The listing builds one solid part. Answer for the finished solid, in the listing's coordinates (mm). A direction names the side the tool comes from. Give positions to 0.01 mm unless a question says otherwise; leave off trailing zeros. Loops run counter-clockwise (first coordinate to the right, second up) from the corner with the lowest first, then second, coordinate; pieces in that order, holes last. Notation, with made-up numbers: M 80.5,-6.5 L 129.5,-6.5 A31 ccw 129.5,30.5 Z; hole C 65.5,78.25 d8. An arc over 180 degrees is marked long. One line per item, written item: value. Start each with the question number.
Q1. For faces 5 (the flat face through (6.9, 16, 6)), 6 (the cylindrical face through (6.59, 33.89, 6.45)), 7 (the cylindrical face through (6.615, 0.301, 7.056)), determine the directions among +Z, -Z, +X, -X, +Y, -Y from which every point of the face is accessible in a straight line to the end or side of a thin tool.
Q2. A cutting plane is placed at B-B, the plane y = 12. Determine the outline of the cut face in (x, z).
Q3. Consider L1, parallel to Y at x = 20, z = 1; L2, parallel to X at y = 14.5, z = 2.5; L3, parallel to Z at x = 10, y = 4. Determine where each line is inside the solid, lowest interval first.
Q4. A cutting plane is placed at C-C, the plane z = 2.5. Determine the outline of the cut face in (x, y), and give its area (3 significant figures).
Q5. A flat-ended cylindrical pin translates along its axis: pin 1 (5.5 mm diameter, centred on y = 23.5, z = 6, fed in from +X). Find the tip coordinate at first contact, or state that the pin passes through.
Q6. A cutting plane is placed at A-A, the plane x = 20. Determine the outline of the cut face in (y, z).
Q7. A cutting plane is placed at D-D, the plane y = 17.5. Determine the outline of the cut face in (x, z), and give its area (3 significant figures).
Q8. The mould has two halves that part along Y. Classify faces 1 (the cylindrical face through (20, 26, 1)), 2 (the cylindrical face through (20, 14, 1)), 3 (the cylindrical face through (3.627, 36.87, 10.699)), 4 (the flat face through (3, 20, 11)): +Y half, -Y half, draft (parallel to the pull), parting line (faces both ways), or undercut.
from build123d import *

# Parameters (mm, degrees)
F0_W        = 6.9
F0_H        = 40
F1_DEPTH    = 11
F0_W_2      = 23.1
F0_R        = 2
F2_DEPTH    = 3
F3_SIZE     = 6
F4_T1_DEPTH = 11.8208999069
F4_T3_DEPTH = 12.1421356237
F4_T5_DEPTH = 23
F5_SIZE     = 1.5
F6_R        = 1


# Not quite as in the source:
# - a fillet or chamfer that OpenCascade refuses, or shapes differently, is made with other operations: its cross-section is extruded or revolved along the edge and cut away or added


with BuildPart() as f1:
    # F0 (on Top) → F1 (new body)
    with BuildSketch(Plane.XY):
        with Locations((3.45, 20)):
            Rectangle(F0_W, F0_H)
    extrude(amount=F1_DEPTH)

    # F0 (on Top) → F2 (join)
    with BuildSketch(Plane.XY):
        with Locations((18.45, 20)):
            Rectangle(F0_W_2, F0_H)
        with Locations((20, 12)):
            Circle(F0_R, mode=Mode.SUBTRACT)
        with Locations((20, 28)):
            Circle(F0_R, mode=Mode.SUBTRACT)
    extrude(amount=F2_DEPTH)

    # F3
    f3_edges = [f1.edges().sort_by_distance(p)[0] for p in [
        (6.9, 40, 7),
    ]]
    chamfer(f3_edges, length=F3_SIZE)

    # F4: fillet of radius 4 on 4 edges, made by hand

    # F4_s2 → F4_t1 (cut)
    with BuildSketch(Plane.XY.offset(3)):
        with BuildLine():
            ThreePointArc((0, 40), (1.0681383035, 39.602199685), (1.9807136938, 38.9192863062))
            Line((1.9807136938, 38.9192863062), (0.9, 40))
            Line((0.9, 40), (0, 40))
        make_face()
    extrude(amount=F4_T1_DEPTH, mode=Mode.SUBTRACT)

    # F4_s4 → F4_t3 (cut)
    with BuildSketch(Plane.XY.offset(3)):
        with BuildLine():
            ThreePointArc((5.7284271247, 35.1715728753), (6.59551813, 33.87387948), (6.9, 32.3431457505))
            Line((6.9, 32.3431457505), (6.9, 34))
            Line((6.9, 34), (5.7284271247, 35.1715728753))
        make_face()
    extrude(amount=F4_T3_DEPTH, mode=Mode.SUBTRACT)

    # F4_s6 → F4_t5 (cut)
    with BuildSketch(Plane.XY.offset(-10)):
        with BuildLine():
            ThreePointArc((26, 40), (28.8284271247, 38.8284271247), (30, 36))
            Line((30, 36), (30, 40))
            Line((30, 40), (26, 40))
        make_face()
        with BuildLine():
            ThreePointArc((30, 4), (28.8284271247, 1.1715728753), (26, 0))
            Line((26, 0), (30, 0))
            Line((30, 0), (30, 4))
        make_face()
    extrude(amount=F4_T5_DEPTH, mode=Mode.SUBTRACT)

    # F5
    f5_edges = [f1.edges().sort_by_distance(p)[0] for p in [
        (18, 28, 3),
        (18, 12, 3),
    ]]
    chamfer(f5_edges, length=F5_SIZE)

    # F6
    f6_edges = [f1.edges().sort_by_distance(p)[0] for p in [
        (6.9, 0, 7),
        (6.9, 16.171573, 11),
        (6.595518, 33.873879, 11),
        (3.85457, 37.04543, 11),
        (1.068138, 39.6022, 11),
    ]]
    fillet(f6_edges, radius=F6_R)


solid = f1.part
Answer block:
1. face 5: +Z, +X, +Y, -Y
1. face 6: +Z, +X, +Y
1. face 7: +Z, +X, -Y
2. outline: M 0,0 L 18,0 L 18,1.5 L 16.5,3 L 6.9,3 L 6.9,10 A1 ccw 5.9,11 L 0,11 Z; M 22,0 L 30,0 L 30,3 L 23.5,3 L 22,1.5 Z
3. L1: 0 to 10, 14 to 26, 30 to 40
3. L2: 0 to 18.34, 21.66 to 30
3. L3: 0 to 3
4. outline: M 0,0 L 26,0 A4 ccw 30,4 L 30,36 A4 ccw 26,40 L 0,40 Z; hole C 20,12 d6; hole C 20,28 d6
4. area: 1,140 mm^2
5. pin 1: x = 6.9
6. outline: M 0,0 L 10,0 L 10,1.5 L 8.5,3 L 0,3 Z; M 14,0 L 26,0 L 26,1.5 L 24.5,3 L 15.5,3 L 14,1.5 Z; M 30,0 L 40,0 L 40,3 L 31.5,3 L 30,1.5 Z
7. outline: M 0,0 L 30,0 L 30,3 L 6.9,3 L 6.9,10 A1 ccw 5.9,11 L 0,11 Z
7. area: 145 mm^2
8. face 1: undercut
8. face 2: undercut
8. face 3: +Y half
8. face 4: draft
